Could you check a few things on this model? Use its own coordinates, in mm. A direction names the side the tool comes from. Give positions to 0.01 mm unless a question says otherwise; leave off trailing zeros. Write each loop counter-clockwise with the first axis right and the second up, starting at its lowest first coordinate (ties: lowest second). Pieces come first, ordered by that corner, then holes. Notation, with made-up numbers: M 23.25,27.5 L 54.25,27.5 A33 ccw 54.25,57.5 Z; hole C 4.5,14.25 d3. An arc over 180 degrees is marked long. Answer as a JSON object with one key per item and string values. Group by question number.
```python
from build123d import *

# Parameters (mm, degrees)
BOSS_EXTRUDE1_DEPTH = 107.424


with BuildPart() as part:
    # Sketch2 → Boss-Extrude1 (new body)
    with BuildSketch(Plane.XY):
        with BuildLine():
            Line((-269.284845729, 142.112072029), (-219.284845729, 142.112072029))
            ThreePointArc((-219.284845729, 142.112072029), (-216.401959188, 143.026859037), (-214.573963508, 145.436485952))
            Line((-214.573963508, 145.436485952), (-205.756404805, 170.226904714))
            ThreePointArc((-205.756404805, 170.226904714), (-200.756404805, 173.755345637), (-195.756404805, 170.226904714))
            Line((-195.756404805, 170.226904714), (-186.938846102, 145.436485952))
            ThreePointArc((-186.938846102, 145.436485952), (-185.110850422, 143.026859037), (-182.227963882, 142.112072029))
            Line((-182.227963882, 142.112072029), (-132.227963882, 142.112072029))
            Line((-132.227963882, 142.112072029), (-182.227963882, 102.112072029))
            Line((-182.227963882, 102.112072029), (-219.284845729, 102.112072029))
            Line((-219.284845729, 102.112072029), (-269.284845729, 142.112072029))
        make_face()
    extrude(amount=BOSS_EXTRUDE1_DEPTH)


solid = part.part
```
1) If we section it at B-B, the plane x = -223: List the corners of the cut face in (y, z) for me.
2) Please list where these lines run through material, in increasing order: line 1 along Y through (x, z) = (-181, 66); line 2 along Y through (x, z) = (-137.5, 24); line 3 along X through (y, z) = (134.5, 72.5). Write a range as from..to.
3) If we section it at C-C, the plane y = 154: List the corners of the cut face in (x, z) for me.
4) I'm going to push flat-ended pins straight in: pin 1 (3 mm diameter, centred on x = -148, z = 25.5, fed in from +Y); pin 2 (8 mm diameter, centred on y = 156.5, z = 25, fed in from +X); pin 3 (12 mm diameter, centred on x = -232, z = 18, fed in from -Y). Where does each tip first touch, or does it pass through?
5) For faces 1 (the flat face through (-158, 142.112, 53)), 2 (the flat face through (-200, 102.112, 53)), 3 (the flat face through (-245, 142.112, 53)), which set-ups out of +Z, -Z, +X, -X, +Y, -Y let a thin tool reach every point of the face, with its end or its side?
6) If we section it at A-A, the plane z = 60: List the corners of the cut face in (x, y) for me, plus the area to 3 significant figures.
Taken from the geometry:
{
 "1": {"outline": "M 105.08,0 L 142.11,0 L 142.11,107.42 L 105.08,107.42 Z"},
 "2": {"line 1": "103.09..142.11", "line 2": "137.89..142.11", "line 3": "-259.77..-141.74"},
 "3": {"outline": "M -211.53,0 L -189.98,0 L -189.98,107.42 L -211.53,107.42 Z"},
 "4": {"pin 1": "y = 142.11", "pin 2": "x = -189.45", "pin 3": "y = 107.48"},
 "5": {"face 1": "+Z, -Z, +X, +Y", "face 2": "+Z, -Z, +X, -X, -Y", "face 3": "+Z, -Z, -X, +Y"},
 "6": {"outline": "M -269.28,142.11 L -219.28,102.11 L -182.23,102.11 L -132.23,142.11 L -182.23,142.11 A5 cw -186.94,145.44 L -195.76,170.23 A5.31 ccw -205.76,170.23 L -214.57,145.44 A5 cw -219.28,142.11 Z", "area": "4,070 mm²"}
}
